Geometry check sheet. Reference: the model listing, model coordinates, mm. A direction names the side the tool comes from. Coordinates: 2 decimals unless noted, no trailing zeros. Write each loop counter-clockwise with the first axis right and the second up, starting at its lowest first coordinate (ties: lowest second). Pieces come first, ordered by that corner, then holes. Notation, with made-up numbers: M 71,-18 L 124,-18 A7 ccw 124,-5 Z; hole C 60,22 d1. An arc over 180 degrees is marked long. Write each question's results on one line, items separated by ' | '.
Autodesk Inventor part; units mm, degrees
ref_plane "YZ Plane" through (0, 0, 0) normal (1, 0, 0) x (0, 1, 0)
ref_plane "XZ Plane" through (0, 0, 0) normal (0, 1, 0) x (-1, 0, 0)
ref_plane "XY Plane" through (0, 0, 0) normal (0, 0, 1) x (1, 0, 0)
sketch "Sketch1" plane through (0, 0, 0) normal (0, 0, 1) x (1, 0, 0)
  arc A0 (-1.7105, 10.9635) -> (1.7105, 10.9635) centre (0, 12) ccw
  arc A1 (-1.7105, 10.9635) -> (-4.0726, 11.818) centre (-3.421, 9.9271) ccw
  arc A2 (4.0726, 11.818) -> (1.7105, 10.9635) centre (3.421, 9.9271) ccw
  arc A3 (-6.75, 5.25) -> (-8.75, 3.25) centre (-6.75, 3.25) ccw
  arc A4 (8.75, 3.25) -> (6.75, 5.25) centre (6.75, 3.25) ccw
  arc A5 (-8.75, -3.25) -> (-6.75, -5.25) centre (-6.75, -3.25) ccw
  arc A6 (6.75, -5.25) -> (8.75, -3.25) centre (6.75, -3.25) ccw
  arc A7 (-8.85, 0.6538) -> (-8.85, -0.6538) centre (-7.5, 0) ccw
  arc A8 (8.85, -0.6538) -> (8.85, 0.6538) centre (7.5, 0) ccw
  line L0 (0, 6.25) -> (0, -6.25) construction
  line L1 (8.75, -3.25) -> (8.75, -1.0897)
  line L2 (8.75, 1.0897) -> (8.75, 3.25)
  line L3 (-8.75, 3.25) -> (-8.75, 1.0897)
  line L4 (-8.75, -1.0897) -> (-8.75, -3.25)
  line L5 (-1.5, -7.25) -> (-1.5, -9.8995)
  line L6 (1.5, -7.25) -> (1.5, -9.8995)
  line L7 (-7.5, 0) -> (7.5, 0) construction
  line L8 (-6.75, -5.25) -> (-3.5, -5.25)
  line L9 (3.5, -5.25) -> (6.75, -5.25)
  line L10 (-6.75, 5.25) -> (-6.75, -5.25) construction
  arc A9 (-1.5, -7.25) -> (-3.5, -5.25) centre (-3.5, -7.25) ccw
  arc A10 (3.5, -5.25) -> (1.5, -7.25) centre (3.5, -7.25) ccw
  arc A11 (-4.0726, 11.818) -> (-4.1667, -11.7851) centre (0, 0) ccw
  arc A12 (4.1667, -11.7851) -> (4.0726, 11.818) centre (0, 0) ccw
  arc A13 (-4.1667, -11.7851) -> (-1.5, -9.8995) centre (-3.5, -9.8995) ccw
  arc A14 (1.5, -9.8995) -> (4.1667, -11.7851) centre (3.5, -9.8995) ccw
  line L11 (-1, 7) -> (1, 7)
  line L12 (-2, 6) -> (-2, 6.25)
  line L13 (2, 6) -> (2, 6.25)
  line L14 (6.75, 5.25) -> (3, 5.25)
  line L15 (-3, 5.25) -> (-6.75, 5.25)
  arc A15 (-1, 7) -> (-2, 6) centre (-1, 6) ccw
  arc A16 (2, 6) -> (1, 7) centre (1, 6) ccw
  arc A17 (-3, 5.25) -> (-2, 6.25) centre (-3, 6.25) ccw
  arc A18 (2, 6.25) -> (3, 5.25) centre (3, 6.25) ccw
  arc A19 (-8.85, 0.6538) -> (-8.75, 1.0897) centre (-9.75, 1.0897) ccw
  arc A20 (-8.75, -1.0897) -> (-8.85, -0.6538) centre (-9.75, -1.0897) ccw
  arc A21 (8.75, 1.0897) -> (8.85, 0.6538) centre (9.75, 1.0897) ccw
  arc A22 (8.85, -0.6538) -> (8.75, -1.0897) centre (9.75, -1.0897) ccw
  line L16 (-8.75, 3.25) -> (8.75, 3.25) construction
  point P0 (0, 0)
  point P1 (-8.75, -0.8292)
  point P2 (-8.75, 0.8292)
  point P3 (8.75, 0.8292)
  point P4 (8.75, -0.8292)
  point P5 (-1.5, -12.4097)
  point P6 (1.5, -5.25)
  point P7 (1.5, -12.4097)
  point P8 (-1.5, -5.25)
  point P9 (-6.75, 0)
  point P10 (-2, 7)
  point P11 (2, 7)
  point P12 (0, 7)
  point P13 (0, 3.25)
  point P14 (0, 10)
  dimension "d3" = 4
  dimension "d5" = 2
  dimension "d6" = 2
  dimension "d7" = 3
  dimension "d8" = 3
  dimension "d10" = 15
  dimension "d11" = 3
  dimension "d15" = 2
  dimension "d16" = 2
  dimension "d17" = 2
  dimension "d18" = 7
  dimension "d19" = 4
  dimension "d20" = 10.5
  dimension "d21" = 1
  dimension "d22" = 1
  dimension "d25" = 12
  dimension "d26" = 12.5
  dimension "d27" = 17.5
extrude "Extrusion1" add sketch "Sketch1" along normal blind 6
properties part number "Aft Endcap Middle"
Q1. Sectioned sample at B-B on y = -6.75. Record the cut outline in (x, z).
Geometry check:
outline: M -10.52,0 L -1.56,0 L -1.56,6 L -10.52,6 Z; M 1.56,0 L 10.52,0 L 10.52,6 L 1.56,6 Z
Q2. Scan lines: probe 1 along X at (y, z) = (-1.5, 3.15); probe 2 along Y at (x, z) = (6, 4.6); probe 3 along Y at (x, z) = (7.5, 1.3). Record each from-to range of solid material in increasing order.
Geometry check:
probe 1: x = -12.41 to -8.75, 8.75 to 12.41 | probe 2: y = -10.97 to -5.25, 5.25 to 10.97 | probe 3: y = -10 to -5.1, 5.1 to 10
Q3. Access from +Z, -Z, +X, -X, +Y, -Y to the whole of each face (thin tool, end or side, straight path). Record for faces 1 (the flat face through (-8.75, -2, 3)), 2 (the flat face through (2.6, 5.5, 6)).
Geometry check:
face 1: +Z, -Z | face 2: +Z, +X, -X, +Y, -Y
Q4. Depth check by flat-ended pin: P1, Ø1.1, axis at x = -5.5, z = 3.5, coming from the -Y side; P2, Ø1, axis at x = -4.5, z = 3, coming from the +Y side; P3, Ø1.1, axis at y = 2.5, z = 3.5, coming from the -X side. Enter the tip coordinate at first touch or a pass-through.
Geometry check:
P1: stops at y = -11.48 | P2: stops at y = 11.84 | P3: stops at x = -12.35
Q5. Sectioned sample at D-D on x = -10.25. Record the cut outline in (y, z).
Geometry check:
outline: M -7.15,0 L 7.15,0 L 7.15,6 L -7.15,6 Z
Q6. Mould release check, pull along Y, two halves, no side actions. Record for faces 3 (the cylindrical face through (12.497, 0.266, 2.958)), 4 (the cylindrical face through (-2.759, 11.814, 2.958)), 5 (the cylindrical face through (-8.18, 4.65, 2.96)): pulls with the +Y half, pulls with the -Y half, needs draft (parallel to the pull), parting line crosses it, or undercut.
Geometry check:
face 3: parting line crosses it | face 4: pulls with the +Y half | face 5: undercut
Q7. Sectioned sample at A-A on x = 5.25. Record the cut outline in (y, z).
Geometry check:
outline: M -11.34,0 L -5.25,0 L -5.25,6 L -11.34,6 Z; M 5.25,0 L 11.34,0 L 11.34,6 L 5.25,6 Z
Q8. Sectioned sample at C-C on y = 7.75. Record the cut outline in (x, z).
Geometry check:
outline: M -9.81,0 L 9.81,0 L 9.81,6 L -9.81,6 Z
